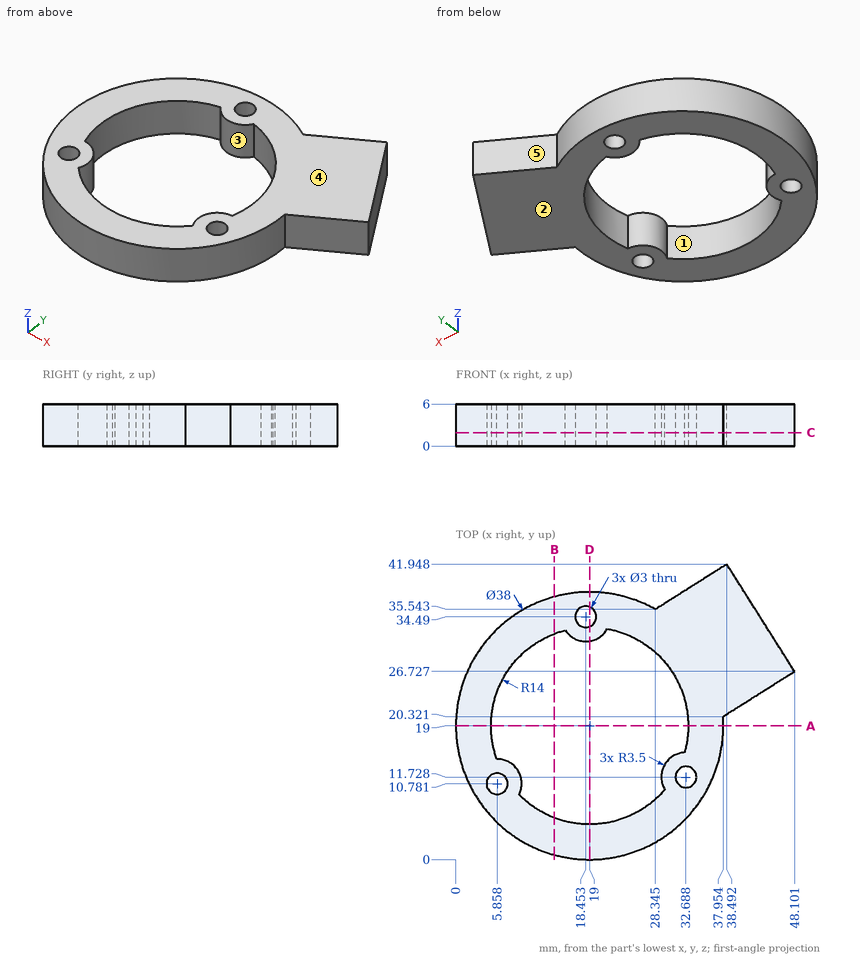
Check sheet for the drawn part. Datum: minimum x, y, z corner. Units: mm. A direction names the side the tool comes from. Give positions to 0.01 mm unless a question says otherwise; leave off trailing zeros. Order: outer loops, then holes, each group sorted by start corner. A loop starts at its lowest first (then second) coordinate and runs counter-clockwise, first axis right, second up. Notation, with made-up numbers: (60.25, -27) -> (78.25, -27) arc R12 ccw to (78.25, -20) -> close; hole circle Ø8 at (-7.75, 81). An arc over 180 degrees is marked (long way). Return JSON: item names as keys, results as strings.
1. Set-up check for the marked faces 1 and 2: record each of +Z, -Z, +X, -X, +Y, -Y from which the full face is reachable in a straight line by a thin tool's end or side.
From the geometry:
{"face 1": "+Z, -Z", "face 2": "-Z, +X, -X, +Y, -Y"}
2. Material ranges on probe 1 along Y at (x, z) = (18.5, 2.4); probe 2 along Y at (x, z) = (6.5, 0.25) (1 decimal); probe 3 along X at (y, z) = (29, 2.2) (1 decimal), recorded low to high. Write a range as [from, to].
From the geometry:
{"probe 1": "[0.01, 5.01], [30.99, 32.99], [35.99, 37.99]", "probe 2": "[4.7, 9.4], [12.1, 14.2], [25.3, 33.3]", "probe 3": "[2.8, 9.2], [28.8, 46.7]"}
3. Cross-section at D-D, the plane x = 19. Record the cut outline in (y, z).
From the geometry:
{"outline": "(0, 0) -> (5, 0) -> (5, 6) -> (0, 6) -> close; (31.03, 0) -> (33.09, 0) -> (33.09, 6) -> (31.03, 6) -> close; (35.89, 0) -> (38, 0) -> (38, 6) -> (35.89, 6) -> close"}
4. Cross-section at A-A, the plane y = 19. Record the cut outline in (x, z).
From the geometry:
{"outline": "(0, 0) -> (5, 0) -> (5, 6) -> (0, 6) -> close; (33, 0) -> (38, 0) -> (38, 6) -> (33, 6) -> close"}
5. Cross-section at C-C, the plane z = 1.95. Record the cut outline in (x, y) (1 decimal).
From the geometry:
{"outline": "(28.3, 35.5) arc R19 ccw (long way) to (38, 20.3) -> (48.1, 26.7) -> (38.5, 41.9) -> close; hole circle Ø3 at (5.9, 10.8); hole (5.8, 14.3) arc R3.5 cw to (9, 9.2) arc R14 ccw to (29.7, 9.9) arc R3.5 cw to (32.5, 15.2) arc R14 ccw to (21.5, 32.8) arc R3.5 cw to (15.5, 32.6) arc R14 ccw to start; hole circle Ø3 at (18.5, 34.5); hole circle Ø3 at (32.7, 11.7)"}
6. Go/stop test with flat-tipped pins: P1, Ø1, axis at x = 28.5, y = 11, coming from the +Z side (3 decimals); P2, Ø1, axis at x = 13.5, z = 4.5, coming from the +Y side; P3, Ø2, axis at x = 7.5, z = 1, coming from the +Y side (1 decimal); P4, Ø3, axis at x = 42, z = 2, coming from the -Y side. Record where each tip stops, or that it passes through.
From the geometry:
{"P1": "through", "P2": "y = 37.33", "P3": "y = 34.8", "P4": "y = 21.93"}
7. Mould release check, pull along Y, two halves, no side actions. Record for the marked faces 3, 4 and 5: +Y half, -Y half, draft (parallel to the pull), parting line (faces both ways), or undercut.
From the geometry:
{"face 3": "undercut", "face 4": "draft", "face 5": "+Y half"}
8. Cross-section at B-B, the plane x = 14. Record the cut outline in (y, z).
From the geometry:
{"outline": "(0.67, 0) -> (5.92, 0) -> (5.92, 6) -> (0.67, 6) -> close; (32.08, 0) -> (37.33, 0) -> (37.33, 6) -> (32.08, 6) -> close"}
